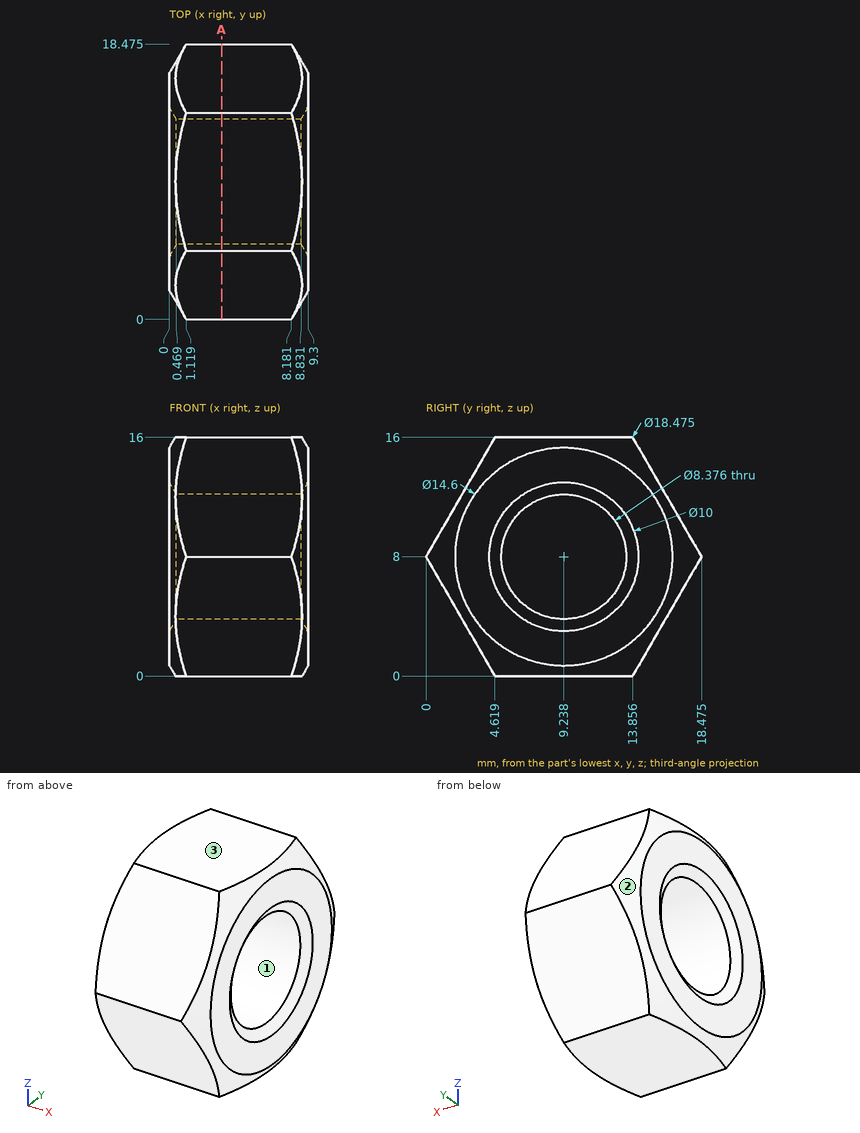
Can you work these out from the drawing? Everything is in mm from the part's minimum corner. Round coordinates to 2 decimals unless told otherwise and drop trailing zeros. Order: outer loops, then holes, each group sorted by start corner. A loop starts at its lowest first (then second) coordinate and runs counter-clockwise, first axis right, second up. Notation, with made-up numbers: M -7.75,37.5 L 9.25,37.5 A36 ccw 9.25,72.5 Z; hole C -32,37.25 d8. An arc over 180 degrees is marked long. One line per question, with ' | ' between items.
1) I want a section at A-A, the plane x = 3.5. Write out the boundary of the cut face in (y, z) (1 decimal), then the cut area to 3 significant figures.
Working result:
outline: M 0,8 L 4.6,0 L 13.9,0 L 18.5,8 L 13.9,16 L 4.6,16 Z; hole C 9.2,8 d8.4 | area: 167 mm²
2) If we mould it in two halves opening along Z, with no side actions, what happens to the marked faces 1, 2 and 3? For each: +Z half, -Z half, draft (parallel to the pull), parting line (faces both ways), or undercut.
Working result:
face 1: undercut | face 2: parting line | face 3: +Z half
3) I need wall thicknesses on line 1 along Z through (x, y) = (7.5, 11.25); line 2 along Z through (x, y) = (4.5, 12); line 3 along Y through (x, z) = (7.5, 7.75) (1 decimal). Which ranges of each line are inside material? Lowest first, please.
Working result:
line 1: 0 to 4.33, 11.67 to 16 | line 2: 0 to 4.85, 11.15 to 16 | line 3: 0.1 to 5.1, 13.4 to 18.3
4) For pin 1 Ø3 at (y, z) = (11, 6.5) entering from -X; pin 2 Ø4 at (x, z) = (4, 2) entering from +Y (1 decimal); pin 3 Ø1 at (x, z) = (2.5, 4) entering from -Y, each with a flat end and sliding along its axis, tell me the tip position at first contact or that it passes through.
Working result:
pin 1: through | pin 2: y = 16.2 | pin 3: y = 2.02
